Verification items for the finished model (mm, model axes). A direction names the side the tool comes from. Coordinates: 2 decimals unless noted, no trailing zeros. Write each loop counter-clockwise with the first axis right and the second up, starting at its lowest first coordinate (ties: lowest second). Pieces come first, ordered by that corner, then holes. Notation, with made-up numbers: (19.5, 18) - (44.5, 18) arc R8 ccw to (44.5, 31) - close; hole circle Ø7 at (-9.5, 16.5). An arc over 180 degrees is marked (long way). Answer as CSV lines item,"result". Start each with the question number.
```python
from build123d import *

# Parameters (mm, degrees)
F1_DEPTH = 25.4
F2_W     = 12.7
F2_H     = 6.604
F3_DEPTH = 25.4
F4_DEPTH = 25.4
F6_DEPTH = 25.4


with BuildPart() as f1:
    # F0 (on Right) → F1 (new body)
    with BuildSketch(Plane.YZ):
        with BuildLine():
            ThreePointArc((-5.499261314, 3.175), (-1.6435009364, -6.1336289969), (6.35, 0))
            ThreePointArc((6.35, 0), (6.1336289969, 1.6435009364), (5.499261314, 3.175))
            Line((5.499261314, 3.175), (0, 3.175))
            Line((0, 3.175), (-5.499261314, 3.175))
        make_face()
    extrude(amount=F1_DEPTH)

    # F2 (on Front) → F3 (cut)
    with BuildSketch(Plane.XZ):
        with Locations((12.7, -3.302)):
            Rectangle(F2_W, F2_H)
    extrude(amount=-F3_DEPTH, mode=Mode.SUBTRACT)

    # F4 (cut): a face of the model
    f4_faces = [f1.faces().sort_by_distance(p)[0] for p in [
        (12.7, 0, -3.175),
    ]]
    extrude(f4_faces, amount=-F4_DEPTH, mode=Mode.SUBTRACT)

    # F5 (on face) → F6 (cut)
    with BuildSketch(Plane(origin=(0, 0, 0), x_dir=(1, 0, 0), z_dir=(0, 0, -1))):
        with BuildLine():
            Line((11.2, 0), (14.2, 0))
            ThreePointArc((14.2, 0), (12.7, 1.5), (11.2, 0))
        make_face()
        with BuildLine():
            ThreePointArc((11.2, 0), (12.7, -1.5), (14.2, 0))
            Line((14.2, 0), (11.2, 0))
        make_face()
    extrude(amount=-F6_DEPTH, mode=Mode.SUBTRACT)


solid = f1.part
```
1. Draft check along X on faces 1 (the face through (13, -2, 3.175)), 2 (the face through (0, 0, 0)), 3 (the face through (25.4, 0, 0)), 4 (the face through (6.35, 0, -3)). Enter one of: pulls with the +X half, pulls with the -X half, needs draft (parallel to the pull), parting line crosses it, or undercut.
2. Scan lines: line 1 along X through (y, z) = (-5.5, -1.75); line 2 along Z through (x, y) = (16.25, 0.25) (3 decimals); line 3 along Y through (x, z) = (20.25, -0.25). Record each from-to range of solid material in increasing order. Write a range as from..to.
3. Cross-section at D-D (z = 1.5). Record the cut outline in (x, y).
4. Depth check by flat-ended pin: P1, Ø4, axis at x = 19, y = 4, coming from the -Z side. Enter the tip coordinate at first touch or a pass-through.
5. Cross-section at C-C (z = -1.5). Record the cut outline in (x, y).
6. Access from +Z, -Z, +X, -X, +Y, -Y to the whole of each face (thin tool, end or side, straight path). Record for faces 5 (the face through (13, 2, 0)), 6 (the face through (11.314, -0.575, 1.565)).
7. Cross-section at A-A (x = 12.7). Record the cut outline in (y, z) (3 decimals).
8. Cross-section at B-B (y = 0). Record the cut outline in (x, z) (3 decimals).
Completed:
1,face 1,"needs draft"
1,face 2,"pulls with the -X half"
1,face 3,"pulls with the +X half"
1,face 4,"undercut"
2,line 1,"x = 0..6.35, 19.05..25.4"
2,line 2,"z = 0..3.175"
2,line 3,"y = -6.35..6.35"
3,outline,"(0, -6.17) - (25.4, -6.17) - (25.4, 6.17) - (0, 6.17) - close; hole circle Ø3 at (12.7, 0)"
4,P1,"stops at z = -6.03"
5,outline,"(0, -6.17) - (6.35, -6.17) - (6.35, 6.17) - (0, 6.17) - close; (19.05, -6.17) - (25.4, -6.17) - (25.4, 6.17) - (19.05, 6.17) - close"
6,face 5,"-Z, +Y, -Y"
6,face 6,"+Z, -Z"
7,outline,"(-6.35, 0) - (-1.5, 0) - (-1.5, 3.175) - (-5.499, 3.175) arc R6.35 ccw to start; (1.5, 0) - (6.35, 0) arc R6.35 ccw to (5.499, 3.175) - (1.5, 3.175) - close"
8,outline,"(0, -6.35) - (6.35, -6.35) - (6.35, 0) - (11.2, 0) - (11.2, 3.175) - (0, 3.175) - close; (14.2, 0) - (19.05, 0) - (19.05, -6.35) - (25.4, -6.35) - (25.4, 3.175) - (14.2, 3.175) - close"
